Geometry check sheet. Reference: drawing and pictorial views, mm from the part's lowest x, y, z. A direction names the side the tool comes from. Give positions to 0.01 mm unless a question says otherwise; leave off trailing zeros. Order: outer loops, then holes, each group sorted by start corner. A loop starts at its lowest first (then second) coordinate and runs counter-clockwise, first axis right, second up. Notation, with made-up numbers: (-0.5, 86) - (5.5, 86) arc R19 cw to (5.5, 93) - close; hole circle Ø4 at (38.5, 33). An arc over 180 degrees is marked (long way). Answer as a JSON object with one key per item and string values.
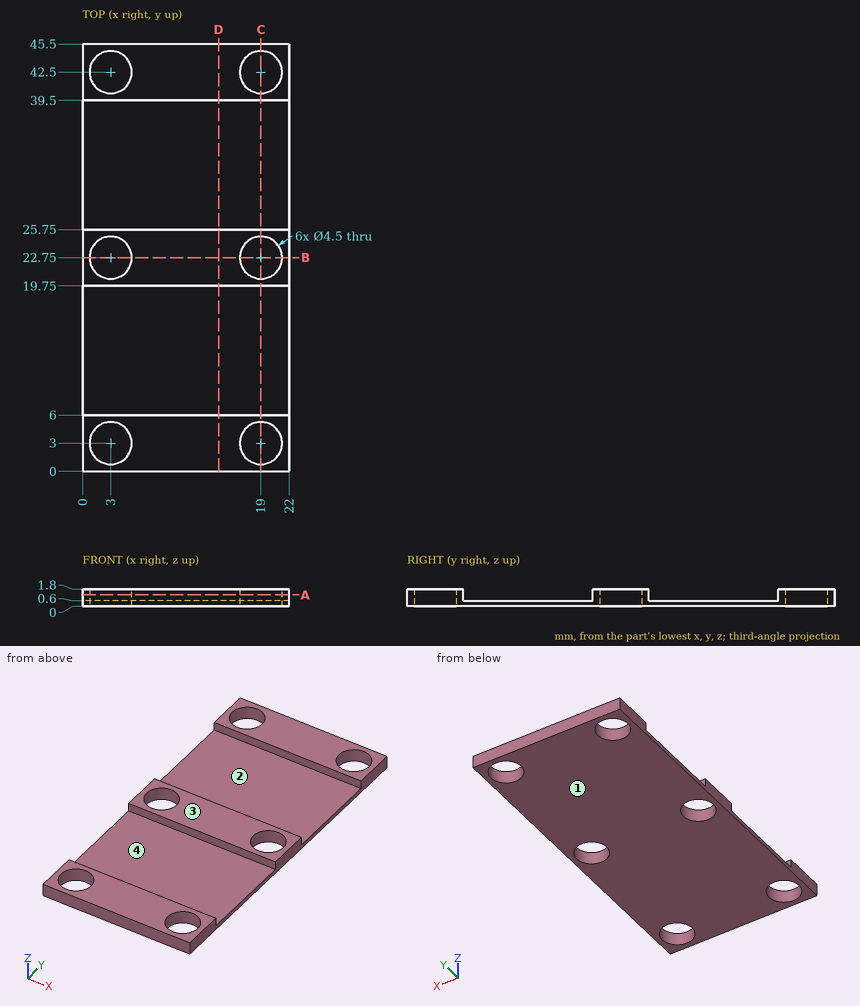
(1) Access from +Z, -Z, +X, -X, +Y, -Y to the whole of each face (thin tool, end or side, straight path). Record for the marked faces 1 and 2.
Computed values:
{"face 1": "-Z, +X, -X, +Y, -Y", "face 2": "+Z, +X, -X"}
(2) Section check D-D (x = 14.5). Record the cut outline in (y, z).
Computed values:
{"outline": "(0, 0) - (45.5, 0) - (45.5, 1.8) - (39.5, 1.8) - (39.5, 0.6) - (25.75, 0.6) - (25.75, 1.8) - (19.75, 1.8) - (19.75, 0.6) - (6, 0.6) - (6, 1.8) - (0, 1.8) - close"}
(3) Section check B-B (y = 22.75). Record the cut outline in (x, z).
Computed values:
{"outline": "(0, 0) - (0.75, 0) - (0.75, 1.8) - (0, 1.8) - close; (5.25, 0) - (16.75, 0) - (16.75, 1.8) - (5.25, 1.8) - close; (21.25, 0) - (22, 0) - (22, 1.8) - (21.25, 1.8) - close"}
(4) Section check A-A (z = 1.2). Count the separate pieces of the cut face and the enclosed holes in it, then the cut area to 3 significant figures.
Computed values:
{"separate pieces": "3", "enclosed holes": "6", "area": "301 mm²"}
(5) Section check C-C (x = 19). Record the cut outline in (y, z).
Computed values:
{"outline": "(0, 0) - (0.75, 0) - (0.75, 1.8) - (0, 1.8) - close; (5.25, 0) - (20.5, 0) - (20.5, 1.8) - (19.75, 1.8) - (19.75, 0.6) - (6, 0.6) - (6, 1.8) - (5.25, 1.8) - close; (25, 0) - (40.25, 0) - (40.25, 1.8) - (39.5, 1.8) - (39.5, 0.6) - (25.75, 0.6) - (25.75, 1.8) - (25, 1.8) - close; (44.75, 0) - (45.5, 0) - (45.5, 1.8) - (44.75, 1.8) - close"}
(6) Material ranges on line 1 along Y through (x, z) = (13.75, 0.95); line 2 along Y through (x, z) = (3, 0.5); line 3 along Y through (x, z) = (3, 1.3), recorded low to high. Write a range as [from, to].
Computed values:
{"line 1": "y = [0, 6], [19.75, 25.75], [39.5, 45.5]", "line 2": "y = [0, 0.75], [5.25, 20.5], [25, 40.25], [44.75, 45.5]", "line 3": "y = [0, 0.75], [5.25, 6], [19.75, 20.5], [25, 25.75], [39.5, 40.25], [44.75, 45.5]"}
(7) Release check for a two-part mould opening along Y. For the marked faces 3 and 4 record: pulls with the +Y half, pulls with the -Y half, needs draft (parallel to the pull), parting line crosses it, or undercut.
Computed values:
{"face 3": "needs draft", "face 4": "undercut"}
(8) Gauge pin test, flat ends, axial feed: pin 1 Ø4 at (x, y) = (3, 22.75) entering from +Z; pin 2 Ø7 at (x, y) = (7, 31) entering from +Z. Record the tip position at first contact, or that the pin passes through.
Computed values:
{"pin 1": "passes through", "pin 2": "stops at z = 0.6"}
